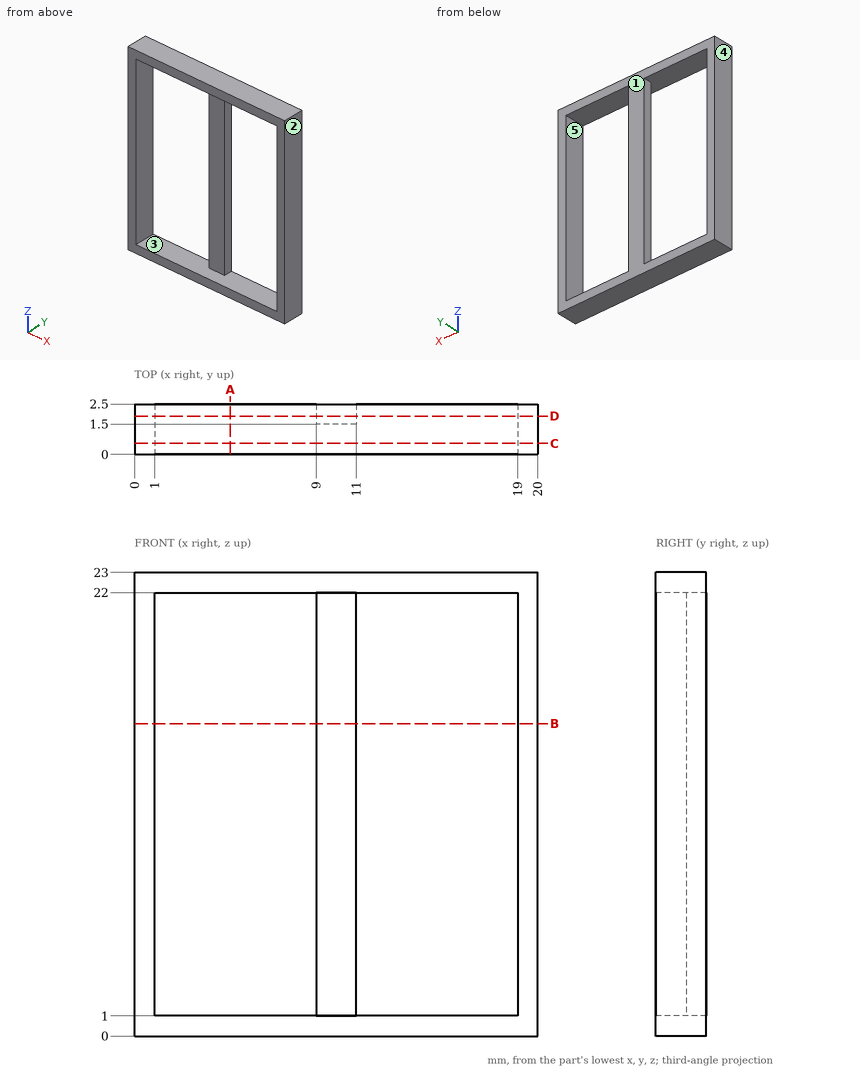
Geometry: see drawing. Coordinates: mm, zero at the bounding-box minimum. A direction names the side the tool comes from. Give positions to 0.01 mm unless a question says otherwise; leave off trailing zeros. Loops run counter-clockwise (first coordinate to the right, second up) from the corner with the lowest first, then second, coordinate; pieces in that order, holes last. Notation, with made-up numbers: (18, -33.5) - (34, -33.5) arc R13 ccw to (34, -26.5) - close; hole circle Ø1 at (-21, -27.75). An arc over 180 degrees is marked (long way). Use CSV: the item, a comma, the result in double quotes. Start each with the question number.
Item 1: Line query: line 1 (X direction, y = 1.9, z = 20.25); line 2 (X direction, y = 0.5, z = 10.75); line 3 (Z direction, x = 13.75, y = 2.45). Output: solid intervals per line, ascending.
Item 2: Mould query, pull axis X, two halves, no side actions, for the marked faces 1, 2 and 3. Classes: pulls with the +X half, pulls with the -X half, needs draft (parallel to the pull), parting line crosses it, or undercut.
Item 3: Section A-A on x = 4.75. Return loops of the section in (y, z), then the cut area to 3 significant figures.
Item 4: Contact query for a flat-ended pin moving along its axis: P1, Ø8, axis at x = 9, z = 15.5, coming from the -Y side. Output: stop coordinate, or through.
Item 5: Reachability of the marked faces 4 and 5 from +Z, -Z, +X, -X, +Y, -Y: full face, straight path, thin tool, end or side. Return the list, or none.
Item 6: Section C-C on y = 0.55. Return loops of the section in (x, z), then the cut area to 3 significant figures.
Item 7: Section D-D on y = 1.9. Return loops of the section in (x, z), then the cut area to 3 significant figures.
Item 8: Section B-B on z = 15.5. Return loops of the section in (x, y), then the cut area to 3 significant figures.
Ans:
1,line 1,"x = 0 to 1, 9 to 11, 19 to 20"
1,line 2,"x = 0 to 1, 19 to 20"
1,line 3,"z = 0 to 1, 22 to 23"
2,face 1,"needs draft"
2,face 2,"pulls with the +X half"
2,face 3,"undercut"
3,outline,"(0, 0) - (2.5, 0) - (2.5, 1) - (0, 1) - close; (0, 22) - (2.5, 22) - (2.5, 23) - (0, 23) - close"
3,area,"5.00 mm2"
4,P1,"stops at y = 1.5"
5,face 4,"+Z, -Z, -X, +Y, -Y"
5,face 5,"+Y, -Y"
6,outline,"(0, 0) - (20, 0) - (20, 23) - (0, 23) - close; hole (1, 1) - (19, 1) - (19, 22) - (1, 22) - close"
6,area,"82.0 mm2"
7,outline,"(0, 0) - (20, 0) - (20, 23) - (0, 23) - close; hole (1, 1) - (9, 1) - (9, 22) - (1, 22) - close; hole (11, 1) - (19, 1) - (19, 22) - (11, 22) - close"
7,area,"124 mm2"
8,outline,"(0, 0) - (1, 0) - (1, 2.5) - (0, 2.5) - close; (9, 1.5) - (11, 1.5) - (11, 2.5) - (9, 2.5) - close; (19, 0) - (20, 0) - (20, 2.5) - (19, 2.5) - close"
8,area,"7.00 mm2"
